Study the drawing (mm; zero at the part's minimum x, y, z) and answer. Round coordinates to 2 decimals unless told otherwise and drop trailing zeros. Loops run counter-clockwise (first coordinate to the right, second up) from the corner with the lowest first, then second, coordinate; pieces in that order, holes last. Notation, with made-up numbers: (-25, 78) -> (22, 78) arc R19 cw to (22, 97) -> close; hole circle Ø5 at (74.5, 50). An arc over 180 degrees is marked (long way). Write each question's results on one line, items separated by ' | '. Start each with the question number.
(1) Straight lines are drawn through the part: probe 1 along Z at (x, y) = (226, 121); probe 2 along X at (y, z) = (152.5, 20); probe 3 along Z at (x, y) = (223, 127). For each, find the intervals that lie inside material, in ascending order.
(2) The part is cut by section A-A (x = 226). Determine the outline of the cut face in (y, z), plus the area to 3 significant figures.
(3) The part is cut by section B-B (z = 16). Determine the outline of the cut face in (x, y), plus the area to 3 significant figures.
(4) A flat-ended cylindrical pin translates along its axis: pin 1 (13 mm diameter, centred on x = 226, z = 16, fed in from +Y). Find the tip coordinate at first contact, or state that the pin passes through.
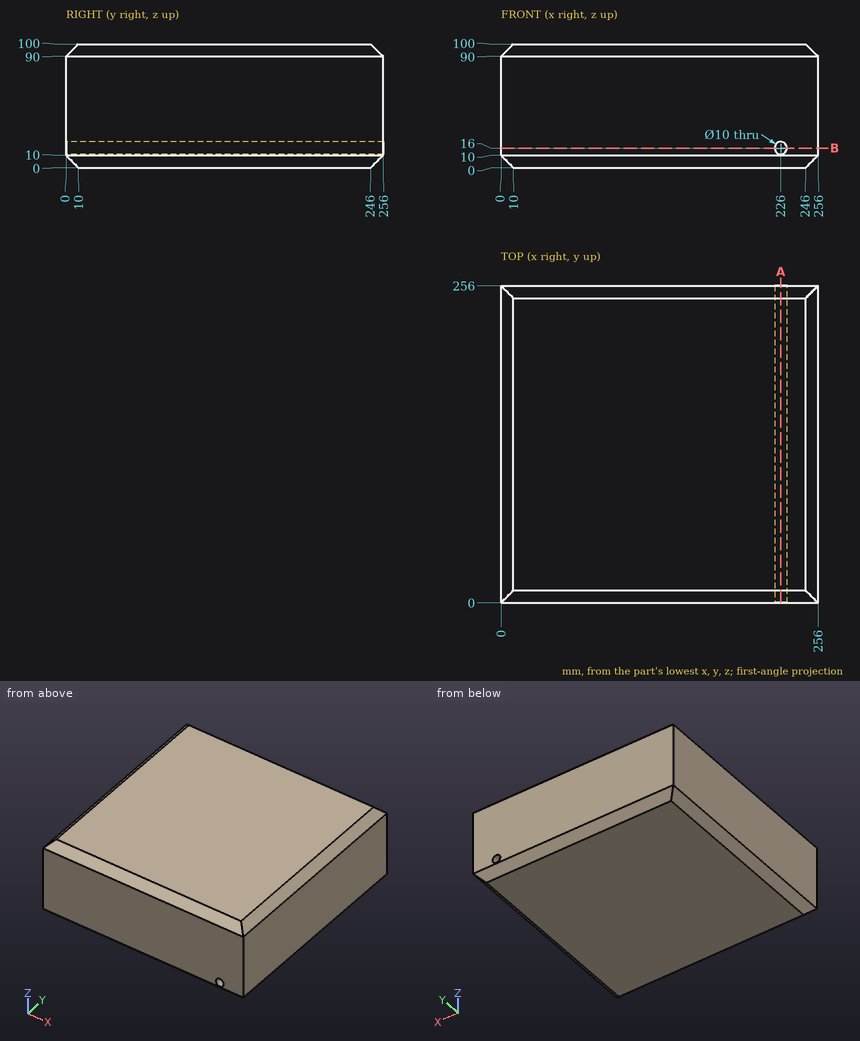
Checked values:
1) probe 1: z = 0 to 11, 21 to 100 | probe 2: x = 0 to 223, 229 to 256 | probe 3: z = 0 to 12, 20 to 100
2) outline: (0, 10) -> (10, 0) -> (246, 0) -> (256, 10) -> (256, 11) -> (0, 11) -> close; (0, 21) -> (256, 21) -> (256, 90) -> (246, 100) -> (10, 100) -> (0, 90) -> close | area: 22,800 mm2
3) outline: (0, 0) -> (221, 0) -> (221, 256) -> (0, 256) -> close; (231, 0) -> (256, 0) -> (256, 256) -> (231, 256) -> close | area: 63,000 mm2
4) pin 1: stops at y = 256
